Build history of the part. All positions in model axes, mm. Face numbers are marked on the shaded views. A direction names the side the tool comes from. Give positions to 0.01 mm unless a question says otherwise; leave off trailing zeros. Order: outer loops, then holes, each group sorted by start corner. A loop starts at its lowest first (then second) coordinate and runs counter-clockwise, first axis right, second up. Notation, with made-up numbers: M -32.5,26 L -21.5,26 A26 cw -21.5,50 Z; hole C 12.25,67.5 d10. An arc over 180 degrees is marked long. One line per item, written item: value. Start each with the question number.
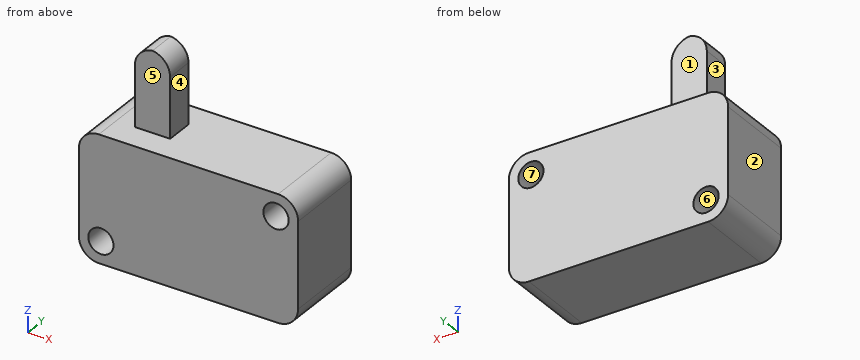
from build123d import *

# Parameters (mm, degrees)
SKETCH1_W           = 27.8
SKETCH1_H           = 15.9
BOSS_EXTRUDE1_DEPTH = 10.3
SKETCH3_R           = 1.6
CUT_EXTRUDE1_DEPTH  = 20.039498418
CIRPATTERN1_COUNT   = 2
BOSS_EXTRUDE2_DEPTH = 10.16
FILLET1_R           = 2.54
FILLET2_R           = 2.54


with BuildPart() as part:
    # Sketch1 → Boss-Extrude1 (new body)
    with BuildSketch(Plane(origin=(0, 0, 0), x_dir=(1, 0, 0), z_dir=(0, 1, 0))):
        Rectangle(SKETCH1_W, SKETCH1_H)
    extrude(amount=BOSS_EXTRUDE1_DEPTH)

    # Sketch3 → Cut-Extrude1 (cut, through all)
    with BuildSketch(Plane(origin=(0, 10.3, 0), x_dir=(1, 0, 0), z_dir=(0, 1, 0))):
        with Locations(Location((-11.1, 5.15, 0), (0, 0, 270))):
            Circle(SKETCH3_R)
    cut_extrude1 = extrude(amount=-CUT_EXTRUDE1_DEPTH, mode=Mode.SUBTRACT)

    # CirPattern1: Cut-Extrude1 ×2 about axis
    cirpattern1_axis = Axis((0, 0, 0), (0, 1, 0))
    for i in range(1, CIRPATTERN1_COUNT):
        add(cut_extrude1.rotate(cirpattern1_axis, i * 360 / CIRPATTERN1_COUNT), mode=Mode.SUBTRACT)

    # Sketch6 → Boss-Extrude2 (add)
    with BuildSketch(Plane.XY.offset(7.95)):
        Polygon((-9, 5.15), (-9, 6.935608094), (-4.523823192, 6.935608094), (-4.523823192, 3.364391906), (-9, 3.364391906), align=None)
    extrude(amount=BOSS_EXTRUDE2_DEPTH)

    # Fillet1
    fillet1_edges = [part.edges().sort_by_distance(p)[0] for p in [
        (13.9, 5.15, 7.95),
        (-13.9, 5.15, 7.95),
        (-13.9, 5.15, -7.95),
        (13.9, 5.15, -7.95),
    ]]
    fillet(fillet1_edges, radius=FILLET1_R)

    # Fillet2
    # the kernel refuses this fillet: 2.54 mm, written as the material it takes off along each edge
    with BuildSketch(Plane(origin=(-9, -2.985608094, 18.11), x_dir=(0, 0, -1), z_dir=(0, 1, 0)), Plane(origin=(-4.523823192, 13.285608094, 18.11), x_dir=(0, 0, -1), z_dir=(0, -1, 0))) as fillet2_piece_1:
        with BuildLine():
            CenterArc((FILLET2_R, -FILLET2_R), FILLET2_R, 90, 90)
            Line((0, -FILLET2_R), (0, 0))
            Line((0, 0), (FILLET2_R, 0))
        make_face()
    extrude(amount=16.271216188, mode=Mode.SUBTRACT)


solid = part.part
1) Drop flat-ended pins along their axis: P1, Ø1.3, axis at x = -7.5, z = 11.5, coming from the +Y side; P2, Ø4, axis at y = 5, z = 12.5, coming from the -X side; P3, Ø2, axis at x = -6.5, z = 15.5, coming from the -Y side; P4, Ø1.9, axis at x = 11.1, z = 5.15, coming from the +Y side. Give the stop position or say it passes through.
2) Slice it at C-C (x = 2.75). List the corners of the cut face in (y, z), plus the area to 3 significant figures.
3) Slice it at A-A (y = 5.25). List the corners of the cut face in (x, z).
4) Tool access for the marked faces 1, 2 and 3: list every direction of +Z, -Z, +X, -X, +Y, -Y with a clear straight run to the whole face (end or side of a thin tool).
5) Pull direction X, two halves, no side cores. Call the marked faces 4, 5, 6 and 7: pulls with the +X half, pulls with the -X half, needs draft (parallel to the pull), parting line crosses it, or undercut.
6) Drill centre lines: line 1 (X direction, y = 7.5, z = -5.15); line 2 (X direction, y = 2.5, z = 5.15); line 3 (X direction, y = 5.5, z = 11). Where is each one in solid material? Low to high.
7) Slice it at D-D (y = 2.5). List the corners of the cut face in (x, z), plus the area to 3 significant figures.
8) Slice it at B-B (z = 6.25). List the corners of the cut face in (x, y), plus the area to 3 significant figures.
Results list:
1. P1: stops at y = 6.94
1. P2: stops at x = -9
1. P3: stops at y = 3.36
1. P4: passes through
2. outline: M 0,-7.95 L 10.3,-7.95 L 10.3,7.95 L 0,7.95 Z
2. area: 164 mm²
3. outline: M -13.9,-5.41 A2.54 ccw -11.36,-7.95 L 11.36,-7.95 A2.54 ccw 13.9,-5.41 L 13.9,5.41 A2.54 ccw 11.36,7.95 L -4.52,7.95 L -4.52,15.57 A2.54 ccw -6.76,18.09 A2.54 ccw -9,15.57 L -9,7.95 L -11.36,7.95 A2.54 ccw -13.9,5.41 Z; hole C -11.1,-5.15 d3.2; hole C 11.1,5.15 d3.2
4. face 1: +Z, +X, -X, +Y
4. face 2: +Z, -Z, -X, +Y, -Y
4. face 3: +Z, -X, +Y, -Y
5. face 4: pulls with the +X half
5. face 5: needs draft
5. face 6: undercut
5. face 7: undercut
6. line 1: x = -13.9 to -12.7, -9.5 to 13.9
6. line 2: x = -13.9 to 9.5, 12.7 to 13.9
6. line 3: x = -9 to -4.52
7. outline: M -13.9,-5.41 A2.54 ccw -11.36,-7.95 L 11.36,-7.95 A2.54 ccw 13.9,-5.41 L 13.9,5.41 A2.54 ccw 11.36,7.95 L -11.36,7.95 A2.54 ccw -13.9,5.41 Z; hole C -11.1,-5.15 d3.2; hole C 11.1,5.15 d3.2
7. area: 420 mm²
8. outline: M -13.76,0 L 9.94,0 L 9.94,10.3 L -13.76,10.3 Z; M 12.26,0 L 13.76,0 L 13.76,10.3 L 12.26,10.3 Z
8. area: 259 mm²
